from build123d import *

# Parameters (mm, degrees)
SKETCH1_W           = 32
SKETCH1_H           = 12.7
BOSS_EXTRUDE1_DEPTH = 12
CUT_EXTRUDE1_DEPTH  = 13.7
SKETCH5_R           = 1.75
CUT_EXTRUDE2_DEPTH  = 6


with BuildPart() as part:
    # Sketch1 → Boss-Extrude1 (new body)
    with BuildSketch(Plane.XY):
        Rectangle(SKETCH1_W, SKETCH1_H)
    extrude(amount=BOSS_EXTRUDE1_DEPTH)

    # Sketch3 → Cut-Revolve1 (revolve, cut)
    with BuildSketch(Plane(origin=(0, 0, 0), x_dir=(0, 0, -1), z_dir=(1, 0, 0))):
        Polygon((0, 6.35), (-8.1, 6.35), (-8.1, 2.65), (-5.8, 2.65), (-5.8, -3.35), (-8.1, -3.35), (-8.1, -6.35), (0, -6.35), align=None)
    revolve(axis=Axis((0, 6.35, 0), (0, -1, 0)), mode=Mode.SUBTRACT)

    # Sketch4 → Cut-Extrude1 (cut, through all)
    with BuildSketch(Plane(origin=(0, 6.35, 0), x_dir=(1, 0, 0), z_dir=(0, 1, 0))):
        with BuildLine():
            Line((-16, -5), (-9.233092656, -5))
            ThreePointArc((-9.233092656, -5), (0, -10.5), (9.233092656, -5))
            Line((9.233092656, -5), (16, -5))
            Line((16, -5), (16, -15))
            Line((16, -15), (-16, -15))
            Line((-16, -15), (-16, -5))
        make_face()
    extrude(amount=-CUT_EXTRUDE1_DEPTH, mode=Mode.SUBTRACT)

    # Sketch5 → Cut-Extrude2 (cut, through all)
    with BuildSketch(Plane.XY.offset(5)):
        with Locations((-13, 0)):
            Circle(SKETCH5_R)
        with Locations((13, 0)):
            Circle(SKETCH5_R)
    extrude(amount=-CUT_EXTRUDE2_DEPTH, mode=Mode.SUBTRACT)


solid = part.part
Verification items for the finished model (mm, model axes). A direction names the side the tool comes from. Round coordinates to 2 decimals unless told otherwise and drop trailing zeros. Write each loop counter-clockwise with the first axis right and the second up, starting at its lowest first coordinate (ties: lowest second). Pieces come first, ordered by that corner, then holes.
(1) Access from +Z, -Z, +X, -X, +Y, -Y to the whole of each face (thin tool, end or side, straight path). Record for faces 5 (the flat face through (-11, 0, 5)), 6 (the flat face through (11, 0, 5)), 7 (the cylindrical face through (0.18, -4.87, 8.1)).
Returned:
face 5: +Z, -X, +Y, -Y
face 6: +Z, +X, +Y, -Y
face 7: -Z, -Y
(2) Section check A-A (y = 0). Enter the section's corners in (x, z).
Returned:
outline: (-16, 0) - (-14.75, 0) - (-14.75, 5) - (-16, 5) - close; (-11.25, 0) - (-5.8, 0) arc R5.8 cw to (5.8, 0) - (11.25, 0) - (11.25, 5) - (9.23, 5) arc R10.5 ccw to (-9.23, 5) - (-11.25, 5) - close; (14.75, 0) - (16, 0) - (16, 5) - (14.75, 5) - close
(3) Section check D-D (y = 4). Enter the section's corners in (x, z).
Returned:
outline: (-16, 0) - (-8.1, 0) arc R8.1 cw to (8.1, 0) - (16, 0) - (16, 5) - (9.23, 5) arc R10.5 ccw to (-9.23, 5) - (-16, 5) - close
(4) Depth check by flat-ended pin: pin 1 Ø1.5 at (x, y) = (12.5, 1) entering from -Z; pin 2 Ø1.5 at (y, z) = (-2.5, 6.5) entering from +X; pin 3 Ø4 at (x, z) = (3, 4) entering from -Y; pin 4 Ø2 at (x, y) = (14, 3) entering from +Z. Enter the tip coordinate at first touch or a pass-through.
Returned:
pin 1: stops at z = 0
pin 2: stops at x = 8.79
pin 3: stops at y = -3.35
pin 4: stops at z = 5
(5) Mould release check, pull along Y, two halves, no side actions. Record for faces 1 (the cylindrical face through (0.18, 4.47, 8.1)), 2 (the cylindrical face through (-11.331, 0.526, 2.535)), 3 (the cylindrical face through (14.669, 0.526, 2.535)), 4 (the flat face through (-2, 2.65, 6)): pulls with the +Y half, pulls with the -Y half, needs draft (parallel to the pull), parting line crosses it, or undercut.
Returned:
face 1: needs draft
face 2: undercut
face 3: undercut
face 4: pulls with the +Y half
(6) Section check C-C (x = 13.5). Enter the section's corners in (y, z).
Returned:
outline: (-6.35, 0) - (-1.68, 0) - (-1.68, 5) - (-6.35, 5) - close; (1.68, 0) - (6.35, 0) - (6.35, 5) - (1.68, 5) - close
(7) Material ranges on line 1 (Y direction, x = -13, z = 1); line 2 (Y direction, x = 12, z = 4.5); line 3 (Z direction, x = 14, y = 2.5), recorded low to high.
Returned:
line 1: y = -6.35 to -1.75, 1.75 to 6.35
line 2: y = -6.35 to -1.44, 1.44 to 6.35
line 3: z = 0 to 5
(8) Section check B-B (z = 1.5). Enter the section's corners in (x, y), plus the area to 3 significant figures.
Returned:
outline: (-16, -6.35) - (-7.96, -6.35) - (-7.96, -3.35) - (-5.6, -3.35) - (-5.6, 2.65) - (-7.96, 2.65) - (-7.96, 6.35) - (-16, 6.35) - close; (5.6, -3.35) - (7.96, -3.35) - (7.96, -6.35) - (16, -6.35) - (16, 6.35) - (7.96, 6.35) - (7.96, 2.65) - (5.6, 2.65) - close; hole circle Ø3.5 at (-13, 0); hole circle Ø3.5 at (13, 0)
area: 213 mm2
